The listing builds one solid part. Answer for the finished solid, in the listing's coordinates (mm). A direction names the side the tool comes from. Coordinates: 2 decimals unless noted, no trailing zeros. Order: outer loops, then holes, each group sorted by start corner. A loop starts at its lowest first (then second) coordinate and runs counter-clockwise, first axis right, second up.
```python
from build123d import *

# Parameters (mm, degrees)
CUT_EXTRUDE1_DEPTH      = 76.150982404
CUT_EXTRUDE1_DEPTH_BACK = 76.150982404
SKETCH2_R               = 4.7625
CHAMFER1_SIZE           = 0.508


with BuildPart() as part:
    # Sketch1 → Revolve1 (revolve)
    with BuildSketch(Plane.XY, mode=Mode.PRIVATE) as revolve1_sk:
        Polygon((-57.15, 6.35), (52.3875, 6.35), (52.3875, 5.9436), (53.3781, 5.9436), (53.3781, 6.35), (55.5625, 6.35), (55.5625, 0), (-74.6125, 0), (-74.6125, 4.7625), (-73.7616, 4.7625), (-73.7616, 4.4704), (-73.025, 4.4704), (-73.025, 4.7625), (-57.15, 4.7625), align=None)
    revolve(revolve1_sk.sketch.rotate(Axis((0, 0, 0), (-1, 0, 0)), 90), axis=Axis((0, 0, 0), (-1, 0, 0)))

    # Sketch2 → Cut-Extrude1 (cut, two sides: drawn at the far end of the back side and taken through both)
    with BuildSketch(Plane.XY.offset(-CUT_EXTRUDE1_DEPTH_BACK)):
        Circle(SKETCH2_R)
    extrude(amount=CUT_EXTRUDE1_DEPTH + CUT_EXTRUDE1_DEPTH_BACK, mode=Mode.SUBTRACT)

    # Chamfer1
    chamfer1_edges = [part.edges().sort_by_distance(p)[0] for p in [
        (-74.6125, 0, 4.7625),
        (55.5625, 0, 6.35),
    ]]
    chamfer(chamfer1_edges, length=CHAMFER1_SIZE)


solid = part.part
```
1) Straight lines are drawn through the part: probe 1 along X at (y, z) = (-0.5, -0.75); probe 2 along X at (y, z) = (0, -2.25); probe 3 along X at (y, z) = (5.5, 1.5). For each, find the intervals that lie inside material, in ascending order.
2) A cutting plane is placed at C-C, the plane x = -50.5. Write down the section's boundary in (y, z), plus the area to 3 significant figures.
3) Each of these flat-tipped pins is pushed along its axis until it touches: P1, Ø3, axis at x = -32, z = 4.5, coming from the -Y side; P2, Ø5, axis at x = 2.5, z = -3, coming from the -Y side. Where does it stop, or does it pass through?
4) For faces 5 (the flat face through (55.562, 0, 0)), 6 (the cylindrical face through (-64.98, 4.65, 1.03)), determine the directions among +Z, -Z, +X, -X, +Y, -Y from which every point of the face is accessible in a straight line to the end or side of a thin tool.
5) The mould has two halves that part along X. Classify faces 1 (the cylindrical face through (52.89, -1.785, -5.669)), 2 (the cylindrical face through (-73.93, 4.65, 1.03)), 3 (the cylindrical face through (-73.388, 4.364, 0.969)), 4 (the flat face through (-57.15, -5, 1)): released by +X, released by -X, zero draft, split by the parting line, or undercut.
6) A cutting plane is placed at D-D, the plane x = 0. Write down the section's boundary in (y, z), plus the area to 3 significant figures.
Working result:
1. probe 1: x = -74.61 to -4.74, 4.74 to 55.56
1. probe 2: x = -74.61 to -4.76, 4.76 to 55.56
1. probe 3: x = -57.15 to 55.56
2. outline: circle Ø12.7 at (0, 0)
2. area: 127 mm2
3. P1: stops at y = -5.6
3. P2: stops at y = -6.33
4. face 5: +Z, -Z, +X, +Y, -Y
4. face 6: -X
5. face 1: undercut
5. face 2: zero draft
5. face 3: undercut
5. face 4: released by -X
6. outline: (-4.76, -4.2) - (-4.76, 4.2) arc R6.35 ccw to start; (4.76, -4.2) arc R6.35 ccw to (4.76, 4.2) - close
6. area: 18.3 mm2
